The model under review builds one solid part; all positions refer to its coordinate system, in mm. Face numbers are marked on the shaded views. A direction names the side the tool comes from. Give positions to 0.01 mm unless a question says otherwise; leave off trailing zeros. Order: outer loops, then holes, each group sorted by start corner. A loop starts at its lowest first (then second) coordinate and runs counter-clockwise, first axis right, second up. Notation, with made-up numbers: (53.25, 25.5) - (112.25, 25.5) arc R13 cw to (112.25, 38.5) - close; hole circle Ø6 at (82, 51). An arc over 180 degrees is marked (long way). Use CSV: the item, a comma, the result in double quotes.
```python
from build123d import *

# Parameters (mm, degrees)
SKETCH1_R           = 31.75
SKETCH1_R_2         = 9.525
BOSS_EXTRUDE1_DEPTH = 9.652
CUT_EXTRUDE1_DEPTH  = 10.652


with BuildPart() as part:
    # Sketch1 → Boss-Extrude1 (new body)
    with BuildSketch(Plane(origin=(0, 0, 0), x_dir=(1, 0, 0), z_dir=(0, 1, 0))):
        Circle(SKETCH1_R)
        Circle(SKETCH1_R_2, mode=Mode.SUBTRACT)
    extrude(amount=BOSS_EXTRUDE1_DEPTH)

    # Sketch2 → Cut-Extrude1 (cut, through all)
    with BuildSketch(Plane(origin=(0, 9.652, 0), x_dir=(1, 0, 0), z_dir=(0, 1, 0))):
        with BuildLine():
            Line((28.575, 0), (43.782696044, 0))
            Line((43.782696044, 0), (43.782696044, 7.720070601))
            Line((43.782696044, 7.720070601), (28.140881542, 4.961996677))
            ThreePointArc((28.140881542, 4.961996677), (28.466263498, 2.490475349), (28.575, 0))
        make_face()
        with BuildLine():
            Line((28.140881542, -4.961996677), (43.782696044, -7.720070601))
            Line((43.782696044, -7.720070601), (41.14227639, -14.974563976))
            Line((41.14227639, -14.974563976), (26.851716639, -9.773225596))
            ThreePointArc((26.851716639, -9.773225596), (27.601330486, -7.395754214), (28.140881542, -4.961996677))
        make_face()
        with BuildLine():
            Line((24.746675913, -14.2875), (38.501856737, -22.229057351))
            Line((38.501856737, -22.229057351), (33.539491009, -28.142974536))
            Line((33.539491009, -28.142974536), (21.889719962, -18.367655947))
            ThreePointArc((21.889719962, -18.367655947), (23.407269666, -16.389946669), (24.746675913, -14.2875))
        make_face()
        with BuildLine():
            Line((18.367655947, -21.889719962), (28.577125281, -34.05689172))
            Line((28.577125281, -34.05689172), (21.891348022, -37.91692702))
            Line((21.891348022, -37.91692702), (14.2875, -24.746675913))
            ThreePointArc((14.2875, -24.746675913), (16.389946669, -23.407269666), (18.367655947, -21.889719962))
        make_face()
        with BuildLine():
            Line((9.773225596, -26.851716639), (15.205570763, -41.77696232))
            Line((15.205570763, -41.77696232), (7.602785381, -43.117538512))
            Line((7.602785381, -43.117538512), (4.961996677, -28.140881542))
            ThreePointArc((4.961996677, -28.140881542), (7.395754214, -27.601330486), (9.773225596, -26.851716639))
        make_face()
        with BuildLine():
            Line((0, -28.575), (0, -44.458114703))
            Line((0, -44.458114703), (-7.602785381, -43.117538512))
            Line((-7.602785381, -43.117538512), (-4.961996677, -28.140881542))
            ThreePointArc((-4.961996677, -28.140881542), (-2.490475349, -28.466263498), (0, -28.575))
        make_face()
        with BuildLine():
            Line((-9.773225596, -26.851716639), (-15.205570763, -41.77696232))
            Line((-15.205570763, -41.77696232), (-21.891348022, -37.91692702))
            Line((-21.891348022, -37.91692702), (-14.2875, -24.746675913))
            ThreePointArc((-14.2875, -24.746675913), (-12.076316829, -25.897745015), (-9.773225596, -26.851716639))
        make_face()
        with BuildLine():
            Line((-18.367655947, -21.889719962), (-28.577125281, -34.05689172))
            Line((-28.577125281, -34.05689172), (-33.539491009, -28.142974536))
            Line((-33.539491009, -28.142974536), (-21.889719962, -18.367655947))
            ThreePointArc((-21.889719962, -18.367655947), (-20.205576272, -20.205576272), (-18.367655947, -21.889719962))
        make_face()
        with BuildLine():
            Line((-24.746675913, -14.2875), (-38.501856737, -22.229057351))
            Line((-38.501856737, -22.229057351), (-41.14227639, -14.974563976))
            Line((-41.14227639, -14.974563976), (-26.851716639, -9.773225596))
            ThreePointArc((-26.851716639, -9.773225596), (-25.897745015, -12.076316829), (-24.746675913, -14.2875))
        make_face()
        with BuildLine():
            Line((-28.140881542, -4.961996677), (-43.782696044, -7.720070601))
            Line((-43.782696044, -7.720070601), (-43.782696044, 0))
            Line((-43.782696044, 0), (-28.575, 0))
            ThreePointArc((-28.575, 0), (-28.466263498, -2.490475349), (-28.140881542, -4.961996677))
        make_face()
        with BuildLine():
            Line((-28.140881542, 4.961996677), (-43.782696044, 7.720070601))
            Line((-43.782696044, 7.720070601), (-41.14227639, 14.974563976))
            Line((-41.14227639, 14.974563976), (-26.851716639, 9.773225596))
            ThreePointArc((-26.851716639, 9.773225596), (-27.601330486, 7.395754214), (-28.140881542, 4.961996677))
        make_face()
        with BuildLine():
            Line((-24.746675913, 14.2875), (-38.501856737, 22.229057351))
            Line((-38.501856737, 22.229057351), (-33.539491009, 28.142974536))
            Line((-33.539491009, 28.142974536), (-21.889719962, 18.367655947))
            ThreePointArc((-21.889719962, 18.367655947), (-23.407269666, 16.389946669), (-24.746675913, 14.2875))
        make_face()
        with BuildLine():
            Line((-18.367655947, 21.889719962), (-28.577125281, 34.05689172))
            Line((-28.577125281, 34.05689172), (-21.891348022, 37.91692702))
            Line((-21.891348022, 37.91692702), (-14.2875, 24.746675913))
            ThreePointArc((-14.2875, 24.746675913), (-16.389946669, 23.407269666), (-18.367655947, 21.889719962))
        make_face()
        with BuildLine():
            Line((-9.773225596, 26.851716639), (-15.205570763, 41.77696232))
            Line((-15.205570763, 41.77696232), (-7.602785381, 43.117538512))
            Line((-7.602785381, 43.117538512), (-4.961996677, 28.140881542))
            ThreePointArc((-4.961996677, 28.140881542), (-7.395754214, 27.601330486), (-9.773225596, 26.851716639))
        make_face()
        with BuildLine():
            Line((0, 28.575), (0, 44.458114703))
            Line((0, 44.458114703), (7.602785381, 43.117538512))
            Line((7.602785381, 43.117538512), (4.961996677, 28.140881542))
            ThreePointArc((4.961996677, 28.140881542), (2.490475349, 28.466263498), (0, 28.575))
        make_face()
        with BuildLine():
            Line((9.773225596, 26.851716639), (15.205570763, 41.77696232))
            Line((15.205570763, 41.77696232), (21.891348022, 37.91692702))
            Line((21.891348022, 37.91692702), (14.2875, 24.746675913))
            ThreePointArc((14.2875, 24.746675913), (12.076316829, 25.897745015), (9.773225596, 26.851716639))
        make_face()
        with BuildLine():
            Line((18.367655947, 21.889719962), (28.577125281, 34.05689172))
            Line((28.577125281, 34.05689172), (33.539491009, 28.142974536))
            Line((33.539491009, 28.142974536), (21.889719962, 18.367655947))
            ThreePointArc((21.889719962, 18.367655947), (20.205576272, 20.205576272), (18.367655947, 21.889719962))
        make_face()
        with BuildLine():
            Line((24.746675913, 14.2875), (38.501856737, 22.229057351))
            Line((38.501856737, 22.229057351), (41.14227639, 14.974563976))
            Line((41.14227639, 14.974563976), (26.851716639, 9.773225596))
            ThreePointArc((26.851716639, 9.773225596), (25.897745015, 12.076316829), (24.746675913, 14.2875))
        make_face()
    extrude(amount=-CUT_EXTRUDE1_DEPTH, mode=Mode.SUBTRACT)


solid = part.part
```
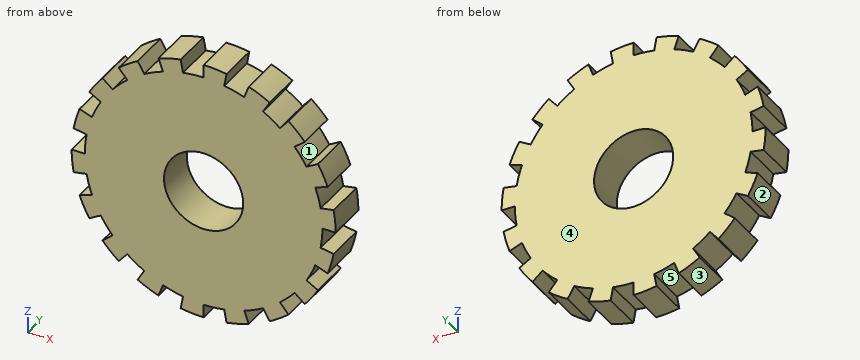
Item 1: Clearance check with flat-ended pins moving along their axes: pin 1 (3.5 mm diameter, centred on x = 29.5, y = 7, fed in from -Z); pin 2 (1.6 mm diameter, centred on x = -30.5, y = 6.5, fed in from +Z); pin 3 (4 mm diameter, centred on x = -7.5, y = 3, fed in from +Z). State where each tip first meets the part, or that it passes through.
Results list:
pin 1,"stops at z = -10.86"
pin 2,"stops at z = 10.86"
pin 3,"stops at z = 31.27"
Item 2: Tool access review of the marked faces 1 and 2: name each direction out of +Z, -Z, +X, -X, +Y, -Y from which nothing blocks a thin tool from reaching the whole face with its end or side.
Results list:
face 1,"+Y, -Y"
face 2,"-Z, -X, +Y, -Y"
Item 3: Take a section at A-A, the plane z = -12. Give the boundary of the cut face in (x, y).
Results list:
outline,"(-29.39, 0) - (25.93, 0) - (25.93, 9.65) - (-29.39, 9.65) - close"
Item 4: Wall thickness on L1, parallel to X at y = 2.25, z = -0.5; L2, parallel to Z at x = -23.5, y = 4; L3, parallel to Z at x = -19, y = 2.25: over which ranges is each line inside the solid? List them lowest first.
Results list:
L1,"x = -31.75 to -9.51, 9.51 to 28.57"
L2,"z = -21.35 to -19.72, -16.26 to 19.72"
L3,"z = -22.64 to 21.34, 22.64 to 25.44"
Item 5: Mouldability with a two-part tool opening along X and no side actions: class the marked faces 3, 4 and 5 as pulls with the +X half, pulls with the -X half, needs draft (parallel to the pull), parting line crosses it, or undercut.
Results list:
face 3,"pulls with the -X half"
face 4,"needs draft"
face 5,"undercut"
